from build123d import *

# Parameters (mm, degrees)
SKETCH1_W           = 316
SKETCH1_H           = 100
BOSS_EXTRUDE1_DEPTH = 10
CUT_EXTRUDE1_REACH  = 168.024
SKETCH4_R           = 3
CUT_EXTRUDE2_REACH  = 168.024
SKETCH5_R           = 2.5
SKETCH6_R           = 4.5
CUT_EXTRUDE3_DEPTH  = 5


with BuildPart() as part:
    # Sketch1 → Boss-Extrude1 (new body)
    with BuildSketch(Plane.XY):
        Rectangle(SKETCH1_W, SKETCH1_H)
    extrude(amount=BOSS_EXTRUDE1_DEPTH)

    # Sketch4 → Cut-Extrude1 (cut, up to next)
    with BuildSketch(Plane(origin=(0, 0, 0), x_dir=(-1, 0, 0), z_dir=(0, 0, -1)), mode=Mode.PRIVATE) as cut_extrude1_sk1:
        with Locations((-138, 30)):
            Circle(SKETCH4_R)
    cut_extrude1_tool1 = extrude(cut_extrude1_sk1.sketch, amount=-CUT_EXTRUDE1_REACH, mode=Mode.PRIVATE) & part.part
    # Sketch4 → Cut-Extrude1 (cut, up to next)
    with BuildSketch(Plane(origin=(0, 0, 0), x_dir=(-1, 0, 0), z_dir=(0, 0, -1)), mode=Mode.PRIVATE) as cut_extrude1_sk2:
        with Locations((-83, 30)):
            Circle(SKETCH4_R)
    cut_extrude1_tool2 = extrude(cut_extrude1_sk2.sketch, amount=-CUT_EXTRUDE1_REACH, mode=Mode.PRIVATE) & part.part
    # Sketch4 → Cut-Extrude1 (cut, up to next)
    with BuildSketch(Plane(origin=(0, 0, 0), x_dir=(-1, 0, 0), z_dir=(0, 0, -1)), mode=Mode.PRIVATE) as cut_extrude1_sk3:
        with Locations((-28, 30)):
            Circle(SKETCH4_R)
    cut_extrude1_tool3 = extrude(cut_extrude1_sk3.sketch, amount=-CUT_EXTRUDE1_REACH, mode=Mode.PRIVATE) & part.part
    # Sketch4 → Cut-Extrude1 (cut, up to next)
    with BuildSketch(Plane(origin=(0, 0, 0), x_dir=(-1, 0, 0), z_dir=(0, 0, -1)), mode=Mode.PRIVATE) as cut_extrude1_sk4:
        with Locations((27, 30)):
            Circle(SKETCH4_R)
    cut_extrude1_tool4 = extrude(cut_extrude1_sk4.sketch, amount=-CUT_EXTRUDE1_REACH, mode=Mode.PRIVATE) & part.part
    # Sketch4 → Cut-Extrude1 (cut, up to next)
    with BuildSketch(Plane(origin=(0, 0, 0), x_dir=(-1, 0, 0), z_dir=(0, 0, -1)), mode=Mode.PRIVATE) as cut_extrude1_sk5:
        with Locations((82, 30)):
            Circle(SKETCH4_R)
    cut_extrude1_tool5 = extrude(cut_extrude1_sk5.sketch, amount=-CUT_EXTRUDE1_REACH, mode=Mode.PRIVATE) & part.part
    # Sketch4 → Cut-Extrude1 (cut, up to next)
    with BuildSketch(Plane(origin=(0, 0, 0), x_dir=(-1, 0, 0), z_dir=(0, 0, -1)), mode=Mode.PRIVATE) as cut_extrude1_sk6:
        with Locations((137, 30)):
            Circle(SKETCH4_R)
    cut_extrude1_tool6 = extrude(cut_extrude1_sk6.sketch, amount=-CUT_EXTRUDE1_REACH, mode=Mode.PRIVATE) & part.part
    # Sketch4 → Cut-Extrude1 (cut, up to next)
    with BuildSketch(Plane(origin=(0, 0, 0), x_dir=(-1, 0, 0), z_dir=(0, 0, -1)), mode=Mode.PRIVATE) as cut_extrude1_sk7:
        with Locations((137, -30)):
            Circle(SKETCH4_R)
    cut_extrude1_tool7 = extrude(cut_extrude1_sk7.sketch, amount=-CUT_EXTRUDE1_REACH, mode=Mode.PRIVATE) & part.part
    # Sketch4 → Cut-Extrude1 (cut, up to next)
    with BuildSketch(Plane(origin=(0, 0, 0), x_dir=(-1, 0, 0), z_dir=(0, 0, -1)), mode=Mode.PRIVATE) as cut_extrude1_sk8:
        with Locations((82, -30)):
            Circle(SKETCH4_R)
    cut_extrude1_tool8 = extrude(cut_extrude1_sk8.sketch, amount=-CUT_EXTRUDE1_REACH, mode=Mode.PRIVATE) & part.part
    # Sketch4 → Cut-Extrude1 (cut, up to next)
    with BuildSketch(Plane(origin=(0, 0, 0), x_dir=(-1, 0, 0), z_dir=(0, 0, -1)), mode=Mode.PRIVATE) as cut_extrude1_sk9:
        with Locations((27, -30)):
            Circle(SKETCH4_R)
    cut_extrude1_tool9 = extrude(cut_extrude1_sk9.sketch, amount=-CUT_EXTRUDE1_REACH, mode=Mode.PRIVATE) & part.part
    # Sketch4 → Cut-Extrude1 (cut, up to next)
    with BuildSketch(Plane(origin=(0, 0, 0), x_dir=(-1, 0, 0), z_dir=(0, 0, -1)), mode=Mode.PRIVATE) as cut_extrude1_sk10:
        with Locations((-28, -30)):
            Circle(SKETCH4_R)
    cut_extrude1_tool10 = extrude(cut_extrude1_sk10.sketch, amount=-CUT_EXTRUDE1_REACH, mode=Mode.PRIVATE) & part.part
    # Sketch4 → Cut-Extrude1 (cut, up to next)
    with BuildSketch(Plane(origin=(0, 0, 0), x_dir=(-1, 0, 0), z_dir=(0, 0, -1)), mode=Mode.PRIVATE) as cut_extrude1_sk11:
        with Locations((-83, -30)):
            Circle(SKETCH4_R)
    cut_extrude1_tool11 = extrude(cut_extrude1_sk11.sketch, amount=-CUT_EXTRUDE1_REACH, mode=Mode.PRIVATE) & part.part
    # Sketch4 → Cut-Extrude1 (cut, up to next)
    with BuildSketch(Plane(origin=(0, 0, 0), x_dir=(-1, 0, 0), z_dir=(0, 0, -1)), mode=Mode.PRIVATE) as cut_extrude1_sk12:
        with Locations((-138, -30)):
            Circle(SKETCH4_R)
    cut_extrude1_tool12 = extrude(cut_extrude1_sk12.sketch, amount=-CUT_EXTRUDE1_REACH, mode=Mode.PRIVATE) & part.part
    add(cut_extrude1_tool1.solids().sort_by_distance((138, 30, 0))[0], mode=Mode.SUBTRACT)
    add(cut_extrude1_tool2.solids().sort_by_distance((83, 30, 0))[0], mode=Mode.SUBTRACT)
    add(cut_extrude1_tool3.solids().sort_by_distance((28, 30, 0))[0], mode=Mode.SUBTRACT)
    add(cut_extrude1_tool4.solids().sort_by_distance((-27, 30, 0))[0], mode=Mode.SUBTRACT)
    add(cut_extrude1_tool5.solids().sort_by_distance((-82, 30, 0))[0], mode=Mode.SUBTRACT)
    add(cut_extrude1_tool6.solids().sort_by_distance((-137, 30, 0))[0], mode=Mode.SUBTRACT)
    add(cut_extrude1_tool7.solids().sort_by_distance((-137, -30, 0))[0], mode=Mode.SUBTRACT)
    add(cut_extrude1_tool8.solids().sort_by_distance((-82, -30, 0))[0], mode=Mode.SUBTRACT)
    add(cut_extrude1_tool9.solids().sort_by_distance((-27, -30, 0))[0], mode=Mode.SUBTRACT)
    add(cut_extrude1_tool10.solids().sort_by_distance((28, -30, 0))[0], mode=Mode.SUBTRACT)
    add(cut_extrude1_tool11.solids().sort_by_distance((83, -30, 0))[0], mode=Mode.SUBTRACT)
    add(cut_extrude1_tool12.solids().sort_by_distance((138, -30, 0))[0], mode=Mode.SUBTRACT)

    # Sketch5 → Cut-Extrude2 (cut, up to next)
    with BuildSketch(Plane.XY.offset(10), mode=Mode.PRIVATE) as cut_extrude2_sk1:
        with Locations((-150.5, -42.5)):
            Circle(SKETCH5_R)
    cut_extrude2_tool1 = extrude(cut_extrude2_sk1.sketch, amount=-CUT_EXTRUDE2_REACH, mode=Mode.PRIVATE) & part.part
    # Sketch5 → Cut-Extrude2 (cut, up to next)
    with BuildSketch(Plane.XY.offset(10), mode=Mode.PRIVATE) as cut_extrude2_sk2:
        with Locations((150.5, -42.5)):
            Circle(SKETCH5_R)
    cut_extrude2_tool2 = extrude(cut_extrude2_sk2.sketch, amount=-CUT_EXTRUDE2_REACH, mode=Mode.PRIVATE) & part.part
    # Sketch5 → Cut-Extrude2 (cut, up to next)
    with BuildSketch(Plane.XY.offset(10), mode=Mode.PRIVATE) as cut_extrude2_sk3:
        with Locations((-150.5, -12.5)):
            Circle(SKETCH5_R)
    cut_extrude2_tool3 = extrude(cut_extrude2_sk3.sketch, amount=-CUT_EXTRUDE2_REACH, mode=Mode.PRIVATE) & part.part
    # Sketch5 → Cut-Extrude2 (cut, up to next)
    with BuildSketch(Plane.XY.offset(10), mode=Mode.PRIVATE) as cut_extrude2_sk4:
        with Locations((150.5, -12.5)):
            Circle(SKETCH5_R)
    cut_extrude2_tool4 = extrude(cut_extrude2_sk4.sketch, amount=-CUT_EXTRUDE2_REACH, mode=Mode.PRIVATE) & part.part
    add(cut_extrude2_tool1.solids().sort_by_distance((-150.5, -42.5, 10))[0], mode=Mode.SUBTRACT)
    add(cut_extrude2_tool2.solids().sort_by_distance((150.5, -42.5, 10))[0], mode=Mode.SUBTRACT)
    add(cut_extrude2_tool3.solids().sort_by_distance((-150.5, -12.5, 10))[0], mode=Mode.SUBTRACT)
    add(cut_extrude2_tool4.solids().sort_by_distance((150.5, -12.5, 10))[0], mode=Mode.SUBTRACT)

    # Sketch6 → Cut-Extrude3 (cut)
    with BuildSketch(Plane(origin=(0, 0, 0), x_dir=(-1, 0, 0), z_dir=(0, 0, -1))):
        with Locations((-150.5, -42.5)):
            Circle(SKETCH6_R)
        with Locations((-150.5, -12.5)):
            Circle(SKETCH6_R)
        with Locations((150.5, -12.5)):
            Circle(SKETCH6_R)
        with Locations((150.5, -42.5)):
            Circle(SKETCH6_R)
    extrude(amount=-CUT_EXTRUDE3_DEPTH, mode=Mode.SUBTRACT)


solid = part.part
Work out the finished part from the listing and answer in its coordinate system (mm). A direction names the side the tool comes from. Round coordinates to 2 decimals unless told otherwise and drop trailing zeros. Write each loop counter-clockwise with the first axis right and the second up, starting at its lowest first coordinate (ties: lowest second). Pieces come first, ordered by that corner, then holes. Notation, with made-up numbers: (68.5, 88.5) - (110.5, 88.5) arc R35 ccw to (110.5, 125.5) - close; hole circle Ø1 at (-25.75, 21.25). An arc over 180 degrees is marked (long way). Answer in a Markdown table with one row per item. Add a question column.
1. A cutting plane is placed at C-C, the plane z = 1.5. Count the separate pieces of the cut face and the enclosed holes in it, and give its area (3 significant figures).
2. Find the intervals of material crossed by line 1 along Y through (x, z) = (-150.5, 6.85); line 2 along Y through (x, z) = (-137, 3); line 3 along X through (y, z) = (-15.5, 3.75), in increasing order. Write a range as from..to.
3. For faces 1 (the cylindrical face through (135.14, -29.1, 4.93)), 2 (the cylindrical face through (146.34, -14.22, 2.46)), determine the directions among +Z, -Z, +X, -X, +Y, -Y from which every point of the face is accessible in a straight line to the end or side of a thin tool.
4. The mould has two halves that part along X. Classify faces 3 (the cylindrical face through (152.81, -13.46, 7.54)), 4 (the flat face through (-158, -1, 5)), 5 (the flat face through (-2, 1, 10)): +X half, -X half, draft (parallel to the pull), parting line (faces both ways), or undercut.
5. Given pin 1 (6.5 mm diameter, centred on x = -150.5, y = -42.5, fed in from -Z), flat-ended and moving along its own axis, determine where the tip first touches the part or whether it passes through.
6. A cutting plane is placed at A-A, the plane x = 28. Determine the outline of the cut face in (y, z).
7. A cutting plane is placed at B-B, the plane y = 30. Determine the outline of the cut face in (x, z).
Worked out:
| question | item | result |
|---|---|---|
| 1 | separate pieces | 1 |
| 1 | enclosed holes | 16 |
| 1 | area | 31,000 mm^2 |
| 2 | line 1 | -50..-45, -40..-15, -10..50 |
| 2 | line 2 | -50..-33, -27..27, 33..50 |
| 2 | line 3 | -158..-153.85, -147.15..147.15, 153.85..158 |
| 3 | face 1 | +Z, -Z |
| 3 | face 2 | -Z |
| 4 | face 3 | undercut |
| 4 | face 4 | -X half |
| 4 | face 5 | draft |
| 5 | pin 1 | z = 5 |
| 6 | outline | (-50, 0) - (-33, 0) - (-33, 10) - (-50, 10) - close; (-27, 0) - (27, 0) - (27, 10) - (-27, 10) - close; (33, 0) - (50, 0) - (50, 10) - (33, 10) - close |
| 7 | outline | (-158, 0) - (-140, 0) - (-140, 10) - (-158, 10) - close; (-134, 0) - (-85, 0) - (-85, 10) - (-134, 10) - close; (-79, 0) - (-30, 0) - (-30, 10) - (-79, 10) - close; (-24, 0) - (25, 0) - (25, 10) - (-24, 10) - close; (31, 0) - (80, 0) - (80, 10) - (31, 10) - close; (86, 0) - (135, 0) - (135, 10) - (86, 10) - close; (141, 0) - (158, 0) - (158, 10) - (141, 10) - close |
